from build123d import *

# Parameters (mm, degrees)
SKETCH1_R           = 3.9878
BOSS_EXTRUDE1_DEPTH = 1.27
SKETCH2_R           = 1.9558
SKETCH2_R_2         = 0.9144
BOSS_EXTRUDE2_DEPTH = 1.27
BOSS_EXTRUDE3_START = 3.4036
SKETCH3_R           = 1.9558
BOSS_EXTRUDE3_DEPTH = 3.4036
SKETCH4_R           = 0.9144
CUT_EXTRUDE1_DEPTH  = 9.193380172


with BuildPart() as part:
    # Sketch1 → Boss-Extrude1 (new body)
    with BuildSketch(Plane.XY):
        Circle(SKETCH1_R)
    extrude(amount=BOSS_EXTRUDE1_DEPTH)

    # Sketch2 → Boss-Extrude2 (add)
    with BuildSketch(Plane.XY.offset(1.27)):
        Circle(SKETCH2_R)
        Circle(SKETCH2_R_2, mode=Mode.SUBTRACT)
    extrude(amount=BOSS_EXTRUDE2_DEPTH)

    # Sketch3 → Boss-Extrude3 (add)
    with BuildSketch(Plane(origin=(0, 0, 0), x_dir=(-1, 0, 0), z_dir=(0, 0, -1)).offset(BOSS_EXTRUDE3_START)):
        with Locations(Location((0, 0, 0), (0, 0, 180))):
            Circle(SKETCH3_R)
    extrude(amount=-BOSS_EXTRUDE3_DEPTH)

    # Sketch4 → Cut-Extrude1 (cut, through all)
    with BuildSketch(Plane(origin=(0, 0, -3.4036), x_dir=(-1, 0, 0), z_dir=(0, 0, -1))):
        Circle(SKETCH4_R)
    extrude(amount=-CUT_EXTRUDE1_DEPTH, mode=Mode.SUBTRACT)


solid = part.part
Input: part model. Units: mm. Frame: model coordinates. A direction names the side the tool comes from. Give positions to 0.01 mm unless a question says otherwise; leave off trailing zeros. Write each loop counter-clockwise with the first axis right and the second up, starting at its lowest first coordinate (ties: lowest second). Pieces come first, ordered by that corner, then holes. Notation, with made-up numbers: (56.25, 65.5) -> (88.25, 65.5) arc R15 cw to (88.25, 91.5) -> close; hole circle Ø4 at (79, -9). An arc over 180 degrees is marked (long way). Use one line per item in the form item = value. Start each with the question number.
1) Ray query, probe 1 along Y at (x, z) = (0, -0.95); probe 2 along Y at (x, z) = (0, 1.1); probe 3 along Z at (x, y) = (2.25, 3). Return the intervals inside material, ascending. Write a range as from..to.
2) Section query D-D on z = 1.05. Return the cut outline in (x, y), then the cut area to 3 significant figures.
3) Section query A-A on y = 0. Return the cut outline in (x, z), then the cut area to 3 significant figures.
4) Set-up query: faces 1 (the cylindrical face through (1.865, 0.587, 1.896)), 2 (the cylindrical face through (3.804, 1.198, 0.626)), 3 (the flat face through (2, 1, 0)). Return all of +Z, -Z, +X, -X, +Y, -Y with unobstructed straight access to the full face (end or side cutting, diameter ignored); none if empty.
5) Section query C-C on z = -0.6. Return the cut outline in (x, y), then the cut area to 3 significant figures.
6) Draft query along Y for faces 4 (the cylindrical face through (0.726, -0.556, -0.473)), 5 (the cylindrical face through (1.865, -0.587, -1.726)), 6 (the flat face through (2, 1, 1.27)). Return one class per face: pulls with the +Y half, pulls with the -Y half, needs draft (parallel to the pull), parting line crosses it, or undercut.
7) Pin query (flat end, axial travel): pin 1 (1 mm diameter, centred on x = 0, z = 2, fed in from +Y); pin 2 (3 mm diameter, centred on y = 2, z = -2, fed in from -X); pin 3 (1.5 mm diameter, centred on x = -1.5, z = -2, fed in from -Y). Return the tip coordinate at first contact, or that it passes through.
Outcome:
q1.probe_1 = -1.96..-0.91, 0.91..1.96
q1.probe_2 = -3.99..-0.91, 0.91..3.99
q1.probe_3 = 0..1.27
q2.outline = circle Ø7.98 at (0, 0); hole circle Ø1.83 at (0, 0)
q2.area = 47.3 mm^2
q3.outline = (-3.99, 0) -> (-1.96, 0) -> (-1.96, -3.4) -> (-0.91, -3.4) -> (-0.91, 2.54) -> (-1.96, 2.54) -> (-1.96, 1.27) -> (-3.99, 1.27) -> close; (0.91, -3.4) -> (1.96, -3.4) -> (1.96, 0) -> (3.99, 0) -> (3.99, 1.27) -> (1.96, 1.27) -> (1.96, 2.54) -> (0.91, 2.54) -> close
q3.area = 17.5 mm^2
q4.face_1 = +Z
q4.face_2 = +Z, -Z
q4.face_3 = -Z
q5.outline = circle Ø3.91 at (0, 0); hole circle Ø1.83 at (0, 0)
q5.area = 9.39 mm^2
q6.face_4 = undercut
q6.face_5 = parting line crosses it
q6.face_6 = needs draft
q7.pin_1 = 1.96
q7.pin_2 = -1.89
q7.pin_3 = -1.81
